Check sheet for the drawn part. Datum: minimum x, y, z corner. Units: mm. Coordinates: 2 decimals unless noted, no trailing zeros. Order: outer loops, then holes, each group sorted by start corner. A loop starts at its lowest first (then second) coordinate and runs counter-clockwise, first axis right, second up.
Q1. Thickness scan on line 1 (Y direction, x = 50.8, z = 18); line 2 (Y direction, x = 50.8, z = 36); line 3 (X direction, y = 31, z = 13). Record the ranges inside material, lowest first.
Q2. Cross-section at C-C, the plane x = 8.5. Record the boundary of the cut face in (y, z).
Q3. Cross-section at D-D, the plane z = 19. Record the boundary of the cut face in (x, y).
Q4. Depth check by flat-ended pin: P1, Ø10, axis at x = 10.5, z = 25.5, coming from the -Y side; P2, Ø5, axis at x = 82, z = 17, coming from the +Y side; P3, Ø2, axis at y = 34, z = 36.5, coming from the +X side. Enter the tip coordinate at first touch or a pass-through.
Q5. Draft check along X on the marked faces 1, 2 and 3. Enter one of: pulls with the +X half, pulls with the -X half, needs draft (parallel to the pull), parting line crosses it, or undercut.
Q6. Cross-section at A-A, the plane y = 50.8. Record the boundary of the cut face in (x, z), and give its area (3 significant figures).
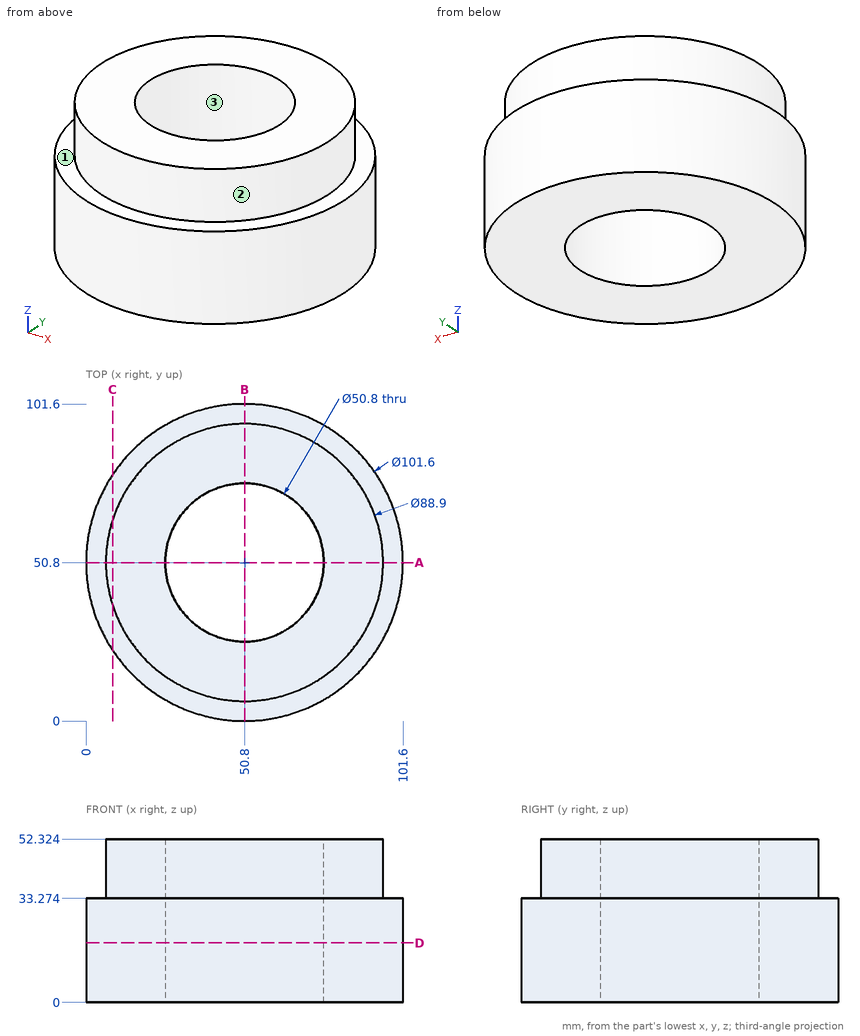
Check values:
1. line 1: y = 0 to 25.4, 76.2 to 101.6
1. line 2: y = 6.35 to 25.4, 76.2 to 95.25
1. line 3: x = 4.02 to 34.89, 66.71 to 97.58
2. outline: (22.67, 0) - (78.93, 0) - (78.93, 33.27) - (64.46, 33.27) - (64.46, 52.32) - (37.14, 52.32) - (37.14, 33.27) - (22.67, 33.27) - close
3. outline: circle Ø101.6 at (50.8, 50.8); hole circle Ø50.8 at (50.8, 50.8)
4. P1: stops at y = 14.27
4. P2: stops at y = 92.72
4. P3: stops at x = 92.35
5. face 1: needs draft
5. face 2: parting line crosses it
5. face 3: undercut
6. outline: (0, 0) - (25.4, 0) - (25.4, 52.32) - (6.35, 52.32) - (6.35, 33.27) - (0, 33.27) - close; (76.2, 0) - (101.6, 0) - (101.6, 33.27) - (95.25, 33.27) - (95.25, 52.32) - (76.2, 52.32) - close
6. area: 2,420 mm2
